Part print with two shaded views. Sizes in mm from the minimum x, y, z corner. A direction names the side the tool comes from. Round coordinates to 2 decimals unless told otherwise and drop trailing zeros. Order: outer loops, then holes, each group sorted by start corner. A loop starts at its lowest first (then second) coordinate and runs counter-clockwise, first axis right, second up. Notation, with made-up numbers: (68, 51.25) -> (116, 51.25) arc R14 cw to (116, 68.25) -> close; hole circle Ø9 at (50, 76.5). An arc over 180 degrees is marked (long way). Put each result on its own line as item: value. Start each with the question number.
Q1. Probe L1, parallel to Z at x = 4.25, y = 6.75; L2, parallel to Y at x = 3.25, z = 5.5; L3, parallel to Y at x = 5.25, z = 3. List the from-to ranges inside material, lowest first.
Q2. Cut at B-B, the plane z = 14.25. List the corners of the cut face in (x, y).
Q3. Cut at C-C, the plane z = 2.75. List the corners of the cut face in (x, y) (1 decimal).
Q4. Flat gauge pins, fed straight in: P1, Ø1, axis at x = 4.5, z = 3.5, coming from the -Y side; P2, Ø3.5, axis at y = 4.5, z = 13, coming from the +X side; P3, Ø1, axis at x = 2.5, z = 13, coming from the -Y side. Where does each tip first touch, or does it go through?
Q5. 3-axis set-ups, long thin cutter, end or side, ignore diameter. For the marked faces 1, 2 and 3: which of +Z, -Z, +X, -X, +Y, -Y reach the whole face in a straight line?
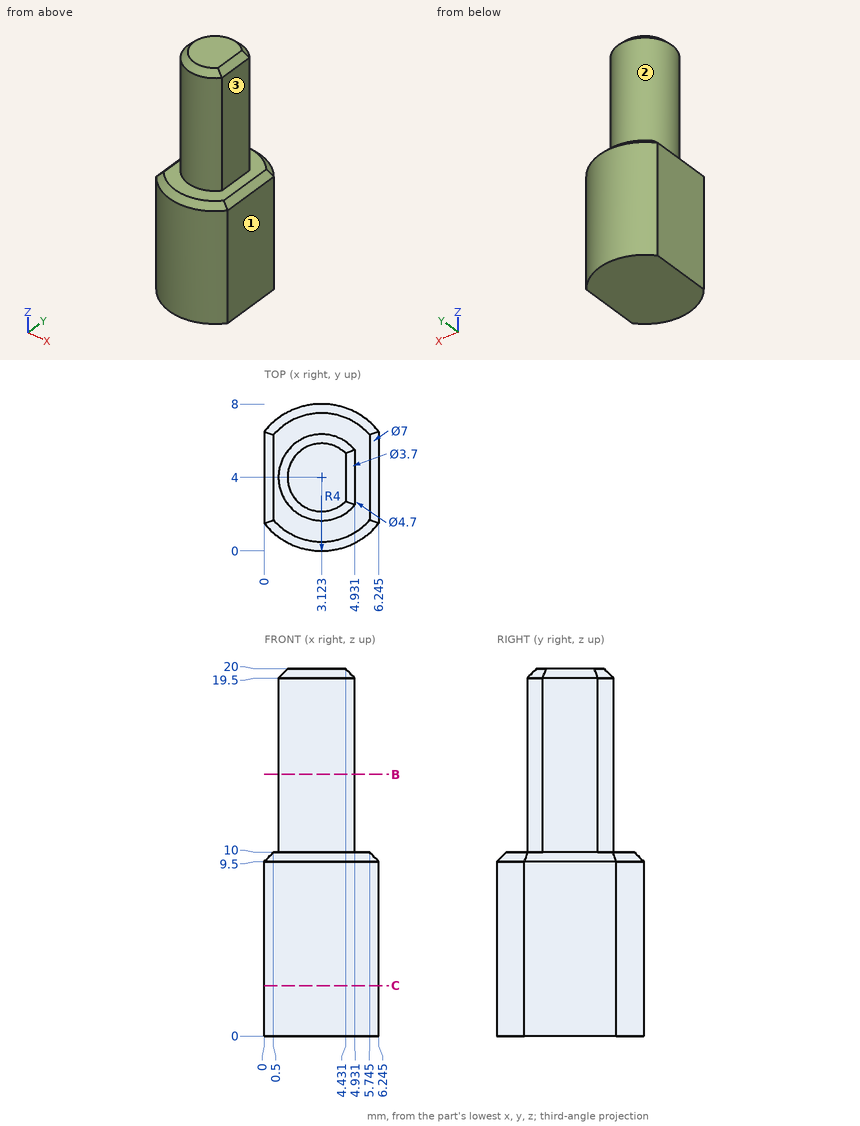
Ans:
1. L1: z = 0 to 10
1. L2: y = 0 to 8
1. L3: y = 0.61 to 7.39
2. outline: (4.93, 2.5) -> (4.93, 5.5) arc R2.35 ccw (long way) to start
3. outline: (0, 1.5) arc R4 ccw to (6.2, 1.5) -> (6.2, 6.5) arc R4 ccw to (0, 6.5) -> close
4. P1: stops at y = 0.1
4. P2: stops at x = 4.93
4. P3: stops at y = 1.65
5. face 1: +Z, -Z, +X, +Y, -Y
5. face 2: +Z
5. face 3: +Z, +X, +Y, -Y
